Could you check a few things on this model? Use its own coordinates, in mm. Face numbers are marked on the shaded views. Coordinates: 2 decimals unless noted, no trailing zeros. Order: outer loops, then holes, each group sorted by start corner. A loop starts at its lowest first (then second) coordinate and runs counter-clockwise, first axis right, second up. Notation, with made-up numbers: (62, 86.25) - (94, 86.25) arc R11 ccw to (94, 92.25) - close; hole circle Ø3 at (20, 23.5). An arc over 180 degrees is marked (long way). Answer as a JSON object with one key per item and string values. Group by question number.
(1) Please list where these lines run through material, in increasing order: probe 1 along Y at (x, z) = (-2.25, 0.2) (3 decimals); probe 2 along Y at (x, z) = (2.75, 0.95); probe 3 along Y at (x, z) = (-4, 0.85).
(2) Imagine slicing it at D-D, the plane y = -6.25. Write out the boundary of the cut face in (x, z), and give its area (3 significant figures).
(3) Imagine slicing it at C-C, the plane z = 0.2. Write out the boundary of the cut face in (x, y).
(4) Imagine slicing it at B-B, the plane x = 3.25. Write out the boundary of the cut face in (y, z), and give its area (3 significant figures).
(5) Imagine slicing it at A-A, the plane y = 0.75. Write out the boundary of the cut face in (x, z), and give its area (3 significant figures).
(6) We'd pull the mould along X, two halves only. Please class the marked faces 1, 2 and 3: pulls with the +X half, pulls with the -X half, needs draft (parallel to the pull), parting line crosses it, or undercut.
(7) Will this pin go through, and if not, where does the flat tip stop? P1, Ø1.7, axis at x = 2.11, y = -6.72, coming from the +Z side.
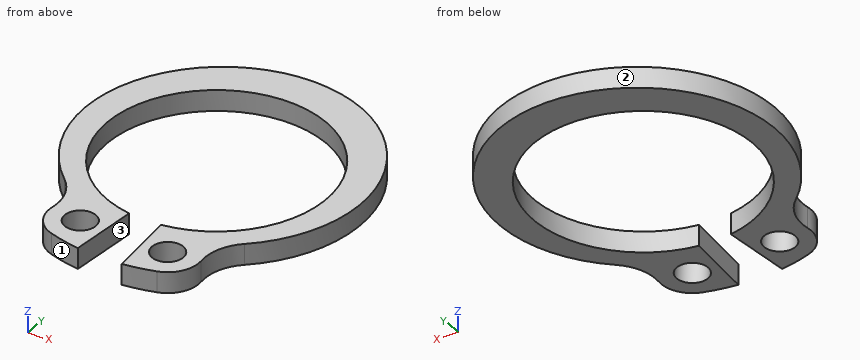
from build123d import *

# Parameters (mm, degrees)
ESQUISSE1_R          = 0.75
BASE_EXTRUSION_DEPTH = 1


with BuildPart() as part:
    # Esquisse1 → Base-Extrusion (new body)
    with BuildSketch(Plane.XY):
        with BuildLine():
            Line((0.768639364, -5.193427917), (1.058921586, -8.480635886))
            ThreePointArc((1.058921586, -8.480635886), (1.81541267, -8.351453574), (2.557265456, -8.154930615))
            ThreePointArc((2.557265456, -8.154930615), (3.375091505, -7.527139269), (3.594515939, -6.519759332))
            ThreePointArc((3.594515939, -6.519759332), (3.716376435, -5.425266349), (4.343048041, -4.519701572))
            ThreePointArc((4.343048041, -4.519701572), (0, 7.05), (-4.343048041, -4.519701572))
            ThreePointArc((-4.343048041, -4.519701572), (-3.716376435, -5.425266349), (-3.594515939, -6.519759332))
            ThreePointArc((-3.594515939, -6.519759332), (-3.375091505, -7.527139269), (-2.557265456, -8.154930615))
            ThreePointArc((-2.557265456, -8.154930615), (-1.81541267, -8.351453574), (-1.058921586, -8.480635886))
            Line((-1.058921586, -8.480635886), (-0.768639364, -5.193427917))
            ThreePointArc((-0.768639364, -5.193427917), (0, 5.25), (0.768639364, -5.193427917))
        make_face()
        with Locations((2.108438165, -6.723653541)):
            Circle(ESQUISSE1_R, mode=Mode.SUBTRACT)
        with Locations(Location((-2.108438165, -6.723653541, 0), (0, 0, 180))):
            Circle(ESQUISSE1_R, mode=Mode.SUBTRACT)
    extrude(amount=BASE_EXTRUSION_DEPTH)


solid = part.part
Result set:
{
 "1": {"probe 1": "y = -8.245 to -7.46, -5.987 to -4.743, 4.743 to 6.655", "probe 2": "y = -8.08 to -7.11, -6.34 to -4.47, 4.47 to 6.45", "probe 3": "y = -4.9 to -3.4, 3.4 to 5.7"},
 "2": {"outline": "(-3.57, 0) - (-2.69, 0) - (-2.69, 1) - (-3.57, 1) - close; (-1.53, 0) - (-0.86, 0) - (-0.86, 1) - (-1.53, 1) - close; (0.86, 0) - (1.53, 0) - (1.53, 1) - (0.86, 1) - close; (2.69, 0) - (3.57, 0) - (3.57, 1) - (2.69, 1) - close", "area": "3.10 mm^2"},
 "3": {"outline": "(-4.34, -4.52) arc R2.25 cw to (-3.59, -6.52) arc R1.5 ccw to (-2.56, -8.15) arc R8.55 ccw to (-1.06, -8.48) - (-0.77, -5.19) arc R5.25 cw (long way) to (0.77, -5.19) - (1.06, -8.48) arc R8.55 ccw to (2.56, -8.15) arc R1.5 ccw to (3.59, -6.52) arc R2.25 cw to (4.34, -4.52) arc R6.6 ccw (long way) to start; hole circle Ø1.5 at (-2.11, -6.72); hole circle Ø1.5 at (2.11, -6.72)"},
 "4": {"outline": "(-7.7, 0) - (-4.12, 0) - (-4.12, 1) - (-7.7, 1) - close; (4.12, 0) - (6.19, 0) - (6.19, 1) - (4.12, 1) - close", "area": "5.64 mm^2"},
 "5": {"outline": "(-6.59, 0) - (-5.2, 0) - (-5.2, 1) - (-6.59, 1) - close; (5.2, 0) - (6.59, 0) - (6.59, 1) - (5.2, 1) - close", "area": "2.79 mm^2"},
 "6": {"face 1": "pulls with the -X half", "face 2": "parting line crosses it", "face 3": "undercut"},
 "7": {"P1": "stops at z = 1"}
}
